Geometry: final body of the model. Coordinates: model frame, mm. A direction names the side the tool comes from. Coordinates: 2 decimals unless noted, no trailing zeros. Loops run counter-clockwise (first coordinate to the right, second up) from the corner with the lowest first, then second, coordinate; pieces in that order, holes last. Notation, with made-up numbers: M 33,54.5 L 54,54.5 A32 ccw 54,89.5 Z; hole C 9,-37 d7. An arc over 180 degrees is marked long. Write each question's results on one line, items separated by ' | '. Start each with the question number.
from build123d import *

# Parameters (mm, degrees)
SKETCH_1_R      = 24.95
SKETCH_1_R_2    = 22.25
EXTRUDE_1_DEPTH = 114.5
SKETCH_2_R      = 23.95
SKETCH_2_R_2    = 22.25
EXTRUDE_2_DEPTH = 22
CHAMFER_1_SIZE  = 1
FILLET_1_R      = 1


with BuildPart() as part:
    # 草图1 → 凸台-拉伸1 (new body)
    with BuildSketch(Plane(origin=(0, 0, 0), x_dir=(1, 0, 0), z_dir=(0, 1, 0))):
        with Locations(Location((0, 0, 0), (0, 0, 90))):
            Circle(SKETCH_1_R)
        with Locations(Location((0, 0, 0), (0, 0, 90))):
            Circle(SKETCH_1_R_2, mode=Mode.SUBTRACT)
    extrude(amount=EXTRUDE_1_DEPTH)

    # 草图2 → 凸台-拉伸2 (add)
    with BuildSketch(Plane(origin=(0, 114.5, 0), x_dir=(1, 0, 0), z_dir=(0, 1, 0))):
        with Locations(Location((0, 0, 0), (0, 0, 270))):
            Circle(SKETCH_2_R)
        with Locations(Location((0, 0, 0), (0, 0, 90))):
            Circle(SKETCH_2_R_2, mode=Mode.SUBTRACT)
    extrude(amount=EXTRUDE_2_DEPTH)

    # 倒角1
    chamfer_1_edges = [part.edges().sort_by_distance(p)[0] for p in [
        (0, 0, 22.25),
    ]]
    chamfer(chamfer_1_edges, length=CHAMFER_1_SIZE)

    # 圆角1
    fillet_1_edges = [part.edges().sort_by_distance(p)[0] for p in [
        (0, 0, 23.25),
        (0, 1, 22.25),
    ]]
    fillet(fillet_1_edges, radius=FILLET_1_R)


solid = part.part
Item 1: Set-up query: faces 1 (the cylindrical face through (-21.04, 56.45, -13.41)), 2 (the flat face through (-22.3, 114.5, 9.4)). Return all of +Z, -Z, +X, -X, +Y, -Y with unobstructed straight access to the full face (end or side cutting, diameter ignored); none if empty.
Item 2: Ray query, L1, parallel to X at y = 62, z = 0; L2, parallel to Z at x = 18, y = 92; L3, parallel to X at y = 47, z = 14. Return the intervals inside material, ascending. Write a range as [from, to].
Item 3: Contact query for flat-ended pins moving along their axis: P1, Ø12, axis at x = -16.5, y = 66.5, coming from the +Z side; P2, Ø12, axis at y = 14, z = 19, coming from the +X side; P3, Ø6, axis at y = 22.5, z = 4.5, coming from the -X side; P4, Ø8, axis at x = -15, z = 5.5, coming from the +Y side. Output: stop coordinate, or through.
Item 4: Pull-direction query (X, two-part tool) for faces 3 (the cylindrical face through (-6.683, 68.012, -21.223)), 4 (the flat face through (-19, 0, -15)), 5 (the cylindrical face through (-23.38, 125.35, -5.19)); classes: released by +X, released by -X, zero draft, split by the parting line, or undercut.
Item 5: Section A-A, the plane y = 11.5. Return loops of the section in (x, z).
Solutions:
1) face 1: +Y, -Y | face 2: +Y
2) L1: x = [-24.95, -22.25], [22.25, 24.95] | L2: z = [-17.28, -13.08], [13.08, 17.28] | L3: x = [-20.65, -17.29], [17.29, 20.65]
3) P1: stops at z = 22.63 | P2: stops at x = 21.3 | P3: stops at x = -24.9 | P4: passes through
4) face 3: undercut | face 4: zero draft | face 5: split by the parting line
5) outline: C 0,0 d49.9; hole C 0,0 d44.5
